The figure shows three views and two pictorial views of one solid part (mm, origin at its lowest corner). Answer the questions. A direction names the side the tool comes from. Coordinates: 2 decimals unless noted, no trailing zeros. Write each loop counter-clockwise with the first axis right and the second up, starting at its lowest first coordinate (ties: lowest second). Pieces come first, ordered by that corner, then holes. Notation, with made-up numbers: (61, -32.75) - (91, -32.75) arc R25 cw to (91, -9.75) - close; hole circle Ø5 at (39.5, 51.5). An arc over 180 degrees is marked (long way). Use a Markdown table: item, result. Add a question column.
(1) Given pin 1 Ø4.5 at (x, z) = (7.5, 7.5) entering from +Y; pin 2 Ø2 at (y, z) = (8.5, 6) entering from +X; pin 3 Ø6 at (x, y) = (6.5, 5) entering from -Z; pin 4 Ø1.5 at (x, y) = (4, 3) entering from -Z, each flat-ended and moving along its own axis, determine where each tip first touches the part or whether it passes through.
(2) A tool of negligible diameter and unlimited length cuts with its end or side. For the marked faces 4 and 5, from which of +Z, -Z, +X, -X, +Y, -Y can it reach the whole face along a straight path? Write none if from no direction.
(3) For a pull along Y with two mould halves and no side action, classify the marked faces 1, 2 and 3 as released by +Y, released by -Y, zero draft, split by the parting line, or undercut.
(4) The part is cut by section D-D, the plane z = 3.25. Give the vertices of the cut face in (x, y), then the cut area to 3 significant figures.
(5) Find the intervals of material crossed by line 1 (X direction, y = 4, z = 7.5); line 2 (Y direction, x = 3.5, z = 1.5), in increasing order. Write a range as from..to.
(6) The part is cut by section A-A, the plane x = 7.5. Give the vertices of the cut face in (y, z).
(7) The part is cut by section B-B, the plane z = 5.75. Give the vertices of the cut face in (x, y), then the cut area to 3 significant figures.
(8) The part is cut by section C-C, the plane y = 9. Give the vertices of the cut face in (x, z).
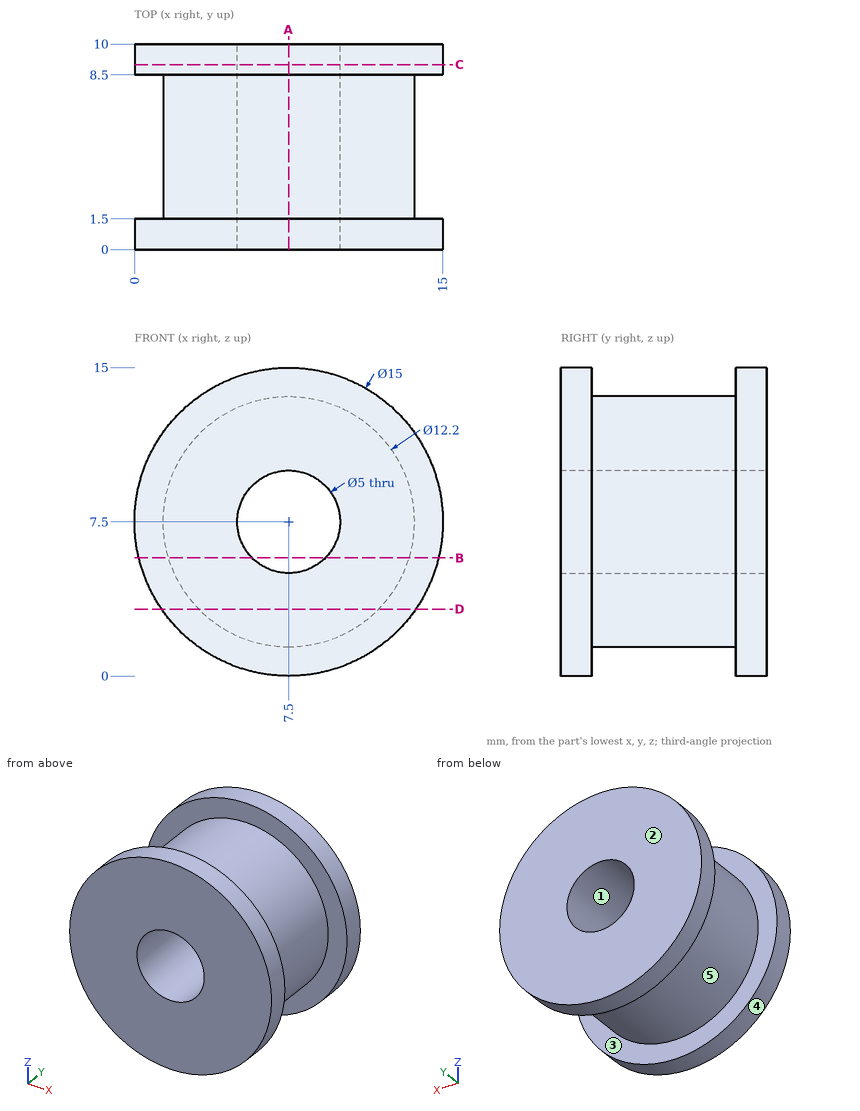
Model answer:
| question | item | result |
|---|---|---|
| 1 | pin 1 | through |
| 1 | pin 2 | x = 14.98 |
| 1 | pin 3 | z = 1.4 |
| 1 | pin 4 | z = 2.06 |
| 2 | face 4 | +Y, -Y |
| 2 | face 5 | none |
| 3 | face 1 | zero draft |
| 3 | face 2 | released by +Y |
| 3 | face 3 | undercut |
| 4 | outline | (1.32, 0) - (13.68, 0) - (13.68, 1.5) - (11.88, 1.5) - (11.88, 8.5) - (13.68, 8.5) - (13.68, 10) - (1.32, 10) - (1.32, 8.5) - (3.12, 8.5) - (3.12, 1.5) - (1.32, 1.5) - close |
| 4 | area | 98.3 mm^2 |
| 5 | line 1 | 1.4..5, 10..13.6 |
| 5 | line 2 | 0..1.5, 8.5..10 |
| 6 | outline | (0, 0) - (1.5, 0) - (1.5, 1.4) - (8.5, 1.4) - (8.5, 0) - (10, 0) - (10, 5) - (0, 5) - close; (0, 10) - (10, 10) - (10, 15) - (8.5, 15) - (8.5, 13.6) - (1.5, 13.6) - (1.5, 15) - (0, 15) - close |
| 7 | outline | (0.21, 0) - (5.71, 0) - (5.71, 10) - (0.21, 10) - (0.21, 8.5) - (1.66, 8.5) - (1.66, 1.5) - (0.21, 1.5) - close; (9.29, 0) - (14.79, 0) - (14.79, 1.5) - (13.34, 1.5) - (13.34, 8.5) - (14.79, 8.5) - (14.79, 10) - (9.29, 10) - close |
| 7 | area | 89.9 mm^2 |
| 8 | outline | circle Ø15 at (7.5, 7.5); hole circle Ø5 at (7.5, 7.5) |
